Autodesk Fusion 360 part; units mm, degrees
sketch "Sketch1" plane through (0, 0, 0) normal (0, 0, 1) x (1, 0, 0)
  line L0 (0, 0) -> (55, 0)
  line L1 (0, 0) -> (0, 100)
  line L2 (0, 100) -> (85, 100)
  line L3 (85, 100) -> (85, 30)
  line L4 (85, 30) -> (55, 0)
  dimension "d1" = 55
  dimension "d2" = 100
  dimension "d3" = 85
  dimension "d4" = 70
extrude "Extrude1" add sketch "Sketch1" along normal blind 30
sketch "Sketch2" plane through (0, 0, 30) normal (0, 0, 1) x (-1, 0, 0)
  line L0 (0, 0) -> (-55, 0)
  line L1 (-55, 0) -> (-85, -30)
  line L2 (-85, -30) -> (-85, -100)
  line L3 (-85, -100) -> (0, -100)
  line L4 (0, -100) -> (0, 0)
  line L5 (0, 0) -> (-10, 0)
  line L6 (-10, 0) -> (-10, -20)
  line L7 (0, 0) -> (0, -100)
  line L8 (-85, -100) -> (-85, -90)
  line L9 (-85, -90) -> (-75, -80)
  line L10 (-75, -80) -> (-45, -80)
  line L11 (-45, -80) -> (-45, -50)
  line L12 (-45, -50) -> (-10, -20)
  dimension "d7" = 10
  dimension "d8" = 20
  dimension "d12" = 30
  dimension "d13" = 30
extrude "Extrude2" add sketch "Sketch2" along normal blind 20 contours L0 L2 L3 L4 L5 L6 L7 L8 L9 L10 L11 L12
sketch "Sketch3" plane through (0, 0, 50) normal (0, 0, 1) x (-1, 0, 0)
  line L0 (-85, -100) -> (0, -100)
  line L1 (0, -100) -> (0, 0)
  line L2 (0, 0) -> (-10, 0)
  line L3 (-10, 0) -> (-10, -20)
  line L4 (-10, -20) -> (-45, -50)
  line L5 (-45, -50) -> (-45, -80)
  line L6 (-45, -80) -> (-75, -80)
  line L7 (-75, -80) -> (-85, -90)
  line L8 (-85, -90) -> (-85, -100)
  line L9 (0, -100) -> (0, -80)
  line L10 (0, -80) -> (-75, -80)
  line L11 (-75, -80) -> (-85, -90)
  line L12 (-85, -90) -> (-85, -100)
  line L13 (-85, -100) -> (0, -100)
  dimension "d16" = 20
extrude "Extrude3" add sketch "Sketch3" along normal blind 10 contours L0 L1 L6 L7 L8 L9 L10 L11 L12 L13
sketch "Sketch4" plane through (0, 0, 50) normal (0, 0, 1) x (-1, 0, 0)
  line L0 (-45, -80) -> (0, -80)
  line L1 (0, -80) -> (0, 0)
  line L2 (0, 0) -> (-10, 0)
  line L3 (-10, 0) -> (-10, -20)
  line L4 (-10, -20) -> (-45, -50)
  line L5 (-45, -50) -> (-45, -80)
  line L6 (0, -80) -> (0, -65)
  line L7 (0, -65) -> (-20, -65)
  dimension "d20" = 20
hole "Hole1" at (20, 65, 50) direction (0, 0, -1) diameter 10 depth 50 tip angle 118
sketch "Sketch5" plane through (0, 80, 0) normal (0, -1, 0) x (1, 0, 0)
  line L0 (45, 30) -> (75, 30)
  line L1 (75, 30) -> (75, 60)
  line L2 (75, 60) -> (0, 60)
  line L3 (0, 60) -> (0, 50)
  line L4 (0, 50) -> (45, 50)
  line L5 (45, 50) -> (45, 30)
  line L6 (45, 50) -> (60, 50)
  line L7 (60, 50) -> (60, 45)
  dimension "d24" = 15
  dimension "d25" = 5
hole "Hole2" at (60, 80, 45) direction (0, 1, 0) diameter 10 depth 20 tip angle 118
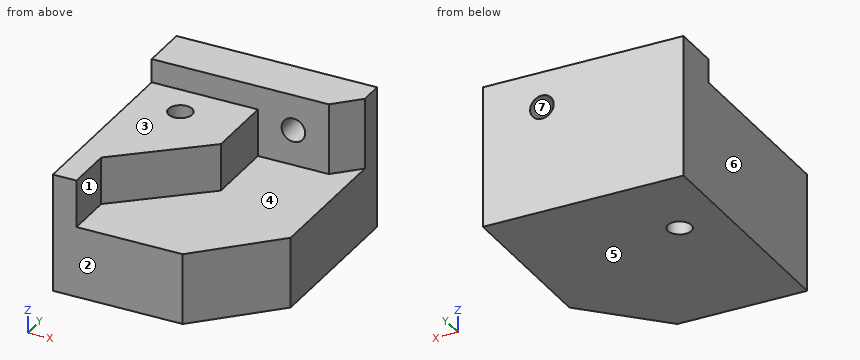
Work out the finished part from the listing and answer in its coordinate system (mm). Face numbers are marked on the shaded views. A direction names the side the tool comes from. Coordinates: 2 decimals unless noted, no trailing zeros. Write each loop counter-clockwise with the first axis right and the second up, starting at its lowest first coordinate (ties: lowest second). Pieces come first, ordered by that corner, then holes. Notation, with made-up numbers: M -28.5,67.5 L -5.5,67.5 A18 ccw -5.5,79.5 Z; hole C 73.5,28 d2. An arc over 180 degrees is marked long. Use one line per item in the form item = value. Start each with the question number.
1. The mould has two halves that part along Z. Classify the marked faces 4, 5, 6 and 7: released by +Z, released by -Z, zero draft, split by the parting line, or undercut.
2. A tool of negligible diameter and unlimited length cuts with its end or side. For the marked faces 1, 2 and 3, from which of +Z, -Z, +X, -X, +Y, -Y can it reach the whole face along a straight path? Write none if from no direction.
3. Straight lines are drawn through the part: probe 1 along Y at (x, z) = (20, 20); probe 2 along Z at (x, y) = (60, 92); probe 3 along Z at (x, y) = (54, 65.5). For each, find the intervals that lie inside material, in ascending order. Write a range as from..to.
4. The part is cut by section B-B (y = 65). Give the vertices of the cut face in (x, z).
5. The part is cut by section D-D (z = 16). Give the vertices of the cut face in (x, y).
6. The part is cut by section C-C (x = 60). Give the vertices of the cut face in (y, z), plus the area to 3 significant figures.
7. Each of these flat-tipped pins is pushed along its axis until it touches: P1, Ø15, axis at x = 26, z = 47.5, coming from the -Y side; P2, Ø1, axis at x = 49.5, z = 34, coming from the -Y side; P3, Ø10, axis at x = 33, y = 11.5, coming from the +Z side; P4, Ø16, axis at x = 60, z = 45, coming from the +Y side. Where does it stop, or does it pass through?
8. The part is cut by section A-A (z = 45). Give the vertices of the cut face in (x, y), plus the area to 3 significant figures.
Evaluation:
q1.face_4 = released by +Z
q1.face_5 = released by -Z
q1.face_6 = zero draft
q1.face_7 = undercut
q2.face_1 = +Z, +X, -Y
q2.face_2 = +Z, -Z, +X, -X, -Y
q2.face_3 = +Z, +X, -X, -Y
q3.probe_1 = 0..60, 70..100
q3.probe_2 = 0..40, 50..60
q3.probe_3 = 0..30
q4.outline = M 0,0 L 15,0 L 15,50 L 0,50 Z; M 25,0 L 85,0 L 85,30 L 45,30 L 45,50 L 25,50 Z
q5.outline = M 0,0 L 55,0 L 85,30 L 85,100 L 0,100 Z; hole C 20,65 d10
q6.outline = M 5,0 L 100,0 L 100,40 L 80,40 L 80,30 L 5,30 Z; M 80,50 L 100,50 L 100,60 L 80,60 Z
q6.area = 3,250 mm^2
q7.P1 = 27.29
q7.P2 = 80
q7.P3 = 30
q7.P4 = 100
q8.outline = M 0,0 L 10,0 L 10,20 L 45,50 L 45,80 L 55,80 L 55,100 L 0,100 Z; M 65,80 L 75,80 L 85,90 L 85,100 L 65,100 Z; hole C 20,65 d10
q8.area = 3,750 mm^2
